The model under review builds one solid part; all positions refer to its coordinate system, in mm. A direction names the side the tool comes from. Coordinates: 2 decimals unless noted, no trailing zeros. Write each loop counter-clockwise with the first axis right and the second up, starting at its lowest first coordinate (ties: lowest second). Pieces come first, ordered by that corner, then holes. Notation, with made-up numbers: (5, -2.75) - (26, -2.75) arc R34 ccw to (26, 34.25) - close; hole circle Ø6 at (37.5, 41.5). An arc over 180 degrees is marked (long way). Put each result on its own line as item: value. Start each with the question number.
Item 1: Consider section A-A on x = 0. Give the boundary of the cut face in (y, z), then the cut area to 3 significant figures.
Item 2: Mouldability with a two-part tool opening along Y and no side actions: class faces 3 (the face through (-6, 0, 1)), 4 (the face through (-0.59, 4.46, 3.05)), 5 (the face through (6, 0, 3.5)) as pulls with the +Y half, pulls with the -Y half, needs draft (parallel to the pull), parting line crosses it, or undercut.
Item 3: For pin 1 (2 mm diameter, centred on y = -2, z = 2.5, fed in from +X); pin 2 (4 mm diameter, centred on x = 2, y = -0.5, fed in from -Z); pin 3 (6.5 mm diameter, centred on x = 0, y = 0, fed in from +Z), all flat-tipped, find the tip position at first contact; note any pin that passes through.
Item 4: To check wall thickness, follow L1, parallel to Y at x = 0, z = 1.35; L2, parallel to Y at x = 0, z = 2.15; L3, parallel to X at y = -1.5, z = 1.35. State the ranges of each line that lie inside material, in increasing order. Write a range as [from, to].
Item 5: Machinability: for faces 1 (the face through (4, -5, 2.7)), 2 (the face through (-1.47, -6.64, 3.11)), which of the approach directions +Z, -Z, +X, -X, +Y, -Y give a long, thin tool a straight path to every point of the face, cutting with its end or side? Answer none if there is none.
Item 6: Consider section C-C on z = 1.05. Give the boundary of the cut face in (x, y).
```python
from build123d import *

# Parameters (mm, degrees)
SKETCH1_R           = 6
SKETCH1_R_2         = 4
BOSS_EXTRUDE1_DEPTH = 3.5
SKETCH4_R           = 5.5
SKETCH4_R_2         = 4.5
CUT_EXTRUDE1_DEPTH  = 41.1
SKETCH6_R           = 0.6
SKETCH8_R           = 6.8
SKETCH8_R_2         = 6
BOSS_EXTRUDE3_DEPTH = 0.8


with BuildPart() as part:
    # Sketch1 → Boss-Extrude1 (new body)
    with BuildSketch(Plane.XY):
        Circle(SKETCH1_R)
        Circle(SKETCH1_R_2, mode=Mode.SUBTRACT)
    extrude(amount=BOSS_EXTRUDE1_DEPTH)

    # Sketch4 → Cut-Extrude1 (cut)
    with BuildSketch(Plane.XY.offset(3.5)):
        Circle(SKETCH4_R)
        Circle(SKETCH4_R_2, mode=Mode.SUBTRACT)
    extrude(amount=-CUT_EXTRUDE1_DEPTH, mode=Mode.SUBTRACT)


with BuildPart() as cut_extrude1_piece_1:
    # of the separate pieces the step leaves, piece 1, a body of its own (cut_extrude1_pieces)
    add(part.part.solids().sort_by_distance((6, 0, 0))[0])



with BuildPart() as cut_extrude1_piece_2:
    # of the separate pieces the step leaves, piece 2, a body of its own (cut_extrude1_pieces)
    add(part.part.solids().sort_by_distance((4.5, 0, 0))[0])


with BuildPart() as cut_extrude1_piece_1_1:
    add(cut_extrude1_piece_1.part)

    add(cut_extrude1_piece_2.part)  # Revolve1 merges Cut-Extrude1 piece 2
    # Sketch6 → Revolve1 (revolve)
    with BuildSketch(Plane(origin=(0, 0, 0), x_dir=(1, 0, 0), z_dir=(0, 1, 0)), mode=Mode.PRIVATE) as revolve1_sk:
        with Locations((-5, -2.265265141)):
            Circle(SKETCH6_R)
    revolve(revolve1_sk.sketch.rotate(Axis((0, 0, 3.5), (0, 0, -1)), 180), axis=Axis((0, 0, 3.5), (0, 0, -1)))

    # Sketch8 → Boss-Extrude3 (add)
    with BuildSketch(Plane.XY.offset(3.5)):
        Circle(SKETCH8_R)
        Circle(SKETCH8_R_2, mode=Mode.SUBTRACT)
    extrude(amount=-BOSS_EXTRUDE3_DEPTH)


solid = cut_extrude1_piece_1_1.part
```
Report:
1. outline: (-6.8, 2.7) - (-6, 2.7) - (-6, 0) - (-5.5, 0) - (-5.5, 1.93) arc R0.6 ccw to (-4.5, 1.93) - (-4.5, 0) - (-4, 0) - (-4, 3.5) - (-4.5, 3.5) - (-4.5, 2.6) arc R0.6 ccw to (-5.5, 2.6) - (-5.5, 3.5) - (-6.8, 3.5) - close; (4, 0) - (4.5, 0) - (4.5, 1.93) arc R0.6 ccw to (5.5, 1.93) - (5.5, 0) - (6, 0) - (6, 2.7) - (6.8, 2.7) - (6.8, 3.5) - (5.5, 3.5) - (5.5, 2.6) arc R0.6 ccw to (4.5, 2.6) - (4.5, 3.5) - (4, 3.5) - close
1. area: 10.4 mm²
2. face 3: parting line crosses it
2. face 4: undercut
2. face 5: needs draft
3. pin 1: x = 6.72
3. pin 2: z = 0
3. pin 3: through
4. L1: [-6, -5.5], [-4.5, -4], [4, 4.5], [5.5, 6]
4. L2: [-6, -4], [4, 6]
4. L3: [-5.81, -5.29], [-4.24, -3.71], [3.71, 4.24], [5.29, 5.81]
5. face 1: -Z
5. face 2: +Z, -Z
6. outline: circle Ø12 at (0, 0); circle Ø9 at (0, 0); hole circle Ø11 at (0, 0); hole circle Ø8 at (0, 0)
